from build123d import *

# Parameters (mm, degrees)
F0_R     = 6.985
F1_DEPTH = 5.08
F2_R     = 6.985
F3_DEPTH = 25.4


with BuildPart() as f1:
    # F0 (on Top) → F1 (new body)
    with BuildSketch(Plane.XY):
        Circle(F0_R)
        with BuildLine():
            ThreePointArc((-2.50952, -2.08153), (-4.59105, 0), (-2.50952, 2.08153))
            Line((-2.50952, 2.08153), (2.50952, 2.08153))
            ThreePointArc((2.50952, 2.08153), (4.59105, 0), (2.50952, -2.08153))
            Line((2.50952, -2.08153), (-2.50952, -2.08153))
        make_face(mode=Mode.SUBTRACT)
    extrude(amount=F1_DEPTH)

    # F2 (on face) → F3 (join)
    with BuildSketch(Plane.XY.offset(5.08)):
        Circle(F2_R)
        with BuildLine():
            ThreePointArc((-5.463988, -1.67513), (0, 5.715), (5.463988, -1.67513))
            Line((5.463988, -1.67513), (5.842, -1.67513))
            Line((5.842, -1.67513), (5.842, -3.204126))
            Line((5.842, -3.204126), (4.732315, -3.204126))
            ThreePointArc((4.732315, -3.204126), (0, -5.715), (-4.732315, -3.204126))
            Line((-4.732315, -3.204126), (-5.842, -3.204126))
            Line((-5.842, -3.204126), (-5.842, -1.67513))
            Line((-5.842, -1.67513), (-5.463988, -1.67513))
        make_face(mode=Mode.SUBTRACT)
    extrude(amount=F3_DEPTH)


solid = f1.part
Here's how the part is built. I have some questions about the finished solid (model axes, mm). A direction names the side the tool comes from. Round coordinates to 2 decimals unless told otherwise and drop trailing zeros. Loops run counter-clockwise (first coordinate to the right, second up) from the corner with the lowest first, then second, coordinate; pieces in that order, holes last. Notation, with made-up numbers: M -2.75,64 L 53.25,64 A16 cw 53.25,80 Z; hole C 63,84 d2. An arc over 180 degrees is marked long. Write each question's results on one line, items separated by ' | '. Start each with the question number.
(1) On a 3-axis mill with a long thin cutter (end or side, diameter ignored), from which of +Z, -Z, +X, -X, +Y, -Y can I reach the whole of each face in a straight line? I mean faces 4 (the flat face through (0, 2.082, 3)), 5 (the flat face through (-5, -3.204, 18)), 6 (the flat face through (0, -3, 0)). Say none if no direction works.
(2) If I drill on probe 1 along Y at (x, z) = (0, 10) (3 decimals); probe 2 along Z at (x, y) = (-0.75, 5.5); probe 3 along Y at (x, z) = (5, 11), over which ranges is the centre line in solid material (lowest first)? Write a range as from..to.
(3) I want a section at C-C (z = 27). Please give me the cut outline in (x, y) (3 decimals).
(4) I want a section at D-D (z = 4). Please give me the cut outline in (x, y) (3 decimals).
(5) Will these pins go through, and if not, where does the flat tip stop? P1, Ø2, axis at x = 1.5, y = 4, coming from the +Z side; P2, Ø0.9, axis at x = 5.5, z = 17, coming from the +Y side; P3, Ø5.5, axis at x = -1, z = 3, coming from the +Y side (3 decimals); P4, Ø0.8, axis at y = -2.5, z = 15.5, coming from the -X side.
(6) I want a section at B-B (y = 0). Please give me the cut outline in (x, z) (3 decimals), then the cut area to 3 significant figures.
(7) Thinking about a two-plate mould opening in Y: for faces 1 (the flat face through (-6, 0, 30.48)), 2 (the cylindrical face through (-0.909, 6.926, 15.027)), 3 (the cylindrical face through (-4.59, -0.05, 2.5)), which applies, pulls with the +Y half, pulls with the -Y half, needs draft (parallel to the pull), parting line crosses it, or undercut?
(8) I want a section at A-A (x = 0). Please give me the cut outline in (y, z) (3 decimals).
Solved:
1) face 4: +Z, -Z | face 5: +Z | face 6: -Z, +X, -X, +Y, -Y
2) probe 1: y = -6.985..-5.715, 5.715..6.985 | probe 2: z = 0..5.08 | probe 3: y = -4.88..-3.2, 2.77..4.88
3) outline: C 0,0 d13.97; hole M -5.842,-3.204 L -4.732,-3.204 A5.715 ccw 4.732,-3.204 L 5.842,-3.204 L 5.842,-1.675 L 5.464,-1.675 A5.715 ccw long -5.464,-1.675 L -5.842,-1.675 Z
4) outline: C 0,0 d13.97; hole M -2.51,-2.082 L 2.51,-2.082 A2.082 ccw 2.51,2.082 L -2.51,2.082 A2.082 ccw Z
5) P1: stops at z = 5.08 | P2: stops at y = 4.83 | P3: stops at y = 6.985 | P4: stops at x = -6.66
6) outline: M -6.985,0 L -4.591,0 L -4.591,5.08 L -5.715,5.08 L -5.715,30.48 L -6.985,30.48 Z; M 4.591,0 L 6.985,0 L 6.985,30.48 L 5.715,30.48 L 5.715,5.08 L 4.591,5.08 Z | area: 88.8 mm²
7) face 1: needs draft | face 2: parting line crosses it | face 3: undercut
8) outline: M -6.985,0 L -2.082,0 L -2.082,5.08 L -5.715,5.08 L -5.715,30.48 L -6.985,30.48 Z; M 2.082,0 L 6.985,0 L 6.985,30.48 L 5.715,30.48 L 5.715,5.08 L 2.082,5.08 Z
